```python
from build123d import *

# Parameters (mm, degrees)
SKETCH1_W            = 12
SKETCH1_H            = 23
BOSS_EXTRUDE1_DEPTH  = 6
SKETCH2_R            = 2.3
SKETCH2_R_2          = 4
CUT_EXTRUDE1_DEPTH   = 6
TAPER_FILLET_SIZE    = 14
TAPER_FILLET_SIZE_2  = 5
TAPER_FILLET2_SIZE   = 14
TAPER_FILLET2_SIZE_2 = 5
EDGE_FILLETS_R       = 1


with BuildPart() as part:
    # Sketch1 → Boss-Extrude1 (new body)
    with BuildSketch(Plane.XY):
        with Locations((6, 11.5)):
            Rectangle(SKETCH1_W, SKETCH1_H)
    extrude(amount=BOSS_EXTRUDE1_DEPTH)

    # Sketch2 → Cut-Extrude1 (cut)
    with BuildSketch(Plane.XY.offset(6)):
        with Locations((6, 18.5)):
            Circle(SKETCH2_R)
        with Locations((6, 6.5)):
            Circle(SKETCH2_R_2)
    extrude(amount=-CUT_EXTRUDE1_DEPTH, mode=Mode.SUBTRACT)

    # taper_fillet
    # an asymmetric fillet: 14, 5 mm, written as the material it takes off along each edge
    with BuildSketch(Plane(origin=(0, 23, -35), x_dir=(0, -1, 0), z_dir=(0, 0, 1))) as taper_fillet_piece_1:
        with BuildLine():
            Bezier((TAPER_FILLET_SIZE, 0), (0, 0), (0, TAPER_FILLET_SIZE_2), weights=[1, 0.707106781, 1])
            Line((0, TAPER_FILLET_SIZE_2), (0, 0))
            Line((0, 0), (TAPER_FILLET_SIZE, 0))
        make_face()
    extrude(amount=76, mode=Mode.SUBTRACT)

    # taper_fillet2
    # an asymmetric fillet: 14, 5 mm, written as the material it takes off along each edge
    with BuildSketch(Plane(origin=(12, 23, -35), x_dir=(0, -1, 0), z_dir=(0, 0, 1))) as taper_fillet2_piece_1:
        with BuildLine():
            Bezier((TAPER_FILLET2_SIZE, 0), (0, 0), (0, -TAPER_FILLET2_SIZE_2), weights=[1, 0.707106781, 1])
            Line((0, -TAPER_FILLET2_SIZE_2), (0, 0))
            Line((0, 0), (TAPER_FILLET2_SIZE, 0))
        make_face()
    extrude(amount=76, mode=Mode.SUBTRACT)

    # edge_fillets
    edge_fillets_edges = [part.edges().sort_by_distance(p)[0] for p in [
        (0, 4.5, 0),
        (0.853211897, 16.822053684, 0),
        (6, 23, 0),
        (12, 4.5, 0),
        (12, 4.5, 6),
        (0, 4.5, 6),
        (0.853211897, 16.822053684, 6),
        (6, 23, 6),
        (0, 0, 3),
        (6, 0, 6),
        (12, 0, 3),
        (6, 0, 0),
        (11.146788103, 16.822053684, 0),
        (11.146788103, 16.822053684, 6),
    ]]
    fillet(edge_fillets_edges, radius=EDGE_FILLETS_R)


solid = part.part
```
Model file for the job. Use its own axes, mm. Round coordinates to 2 decimals unless told otherwise and drop trailing zeros. Write each loop counter-clockwise with the first axis right and the second up, starting at its lowest first coordinate (ties: lowest second). Pieces come first, ordered by that corner, then holes. Notation, with made-up numbers: (87.25, -38.75) - (97.25, -38.75) arc R19 ccw to (97.25, -1.75) - close; hole circle Ø6 at (61.5, 19.25). An arc over 180 degrees is marked (long way). One line per item, written item: value.
(1) Drop a flat-ended pin along its axis: P1, Ø1.5, axis at y = 16, z = 3, coming from the +X side. Give the stop position or say it passes through.
Values follow:
P1: stops at x = 11.47
(2) Cut at B-B, the plane y = 6.5. Give the cut face in (x, z).
Values follow:
outline: (0, 1) arc R1 ccw to (1, 0) - (2, 0) - (2, 6) - (1, 6) arc R1 ccw to (0, 5) - close; (10, 0) - (11, 0) arc R1 ccw to (12, 1) - (12, 5) arc R1 ccw to (11, 6) - (10, 6) - close
(3) Cut at C-C, the plane z = 3. Give the number of separate pieces and of enclosed holes in the cut face, plus the area to 3 significant figures.
Values follow:
separate pieces: 1
enclosed holes: 2
area: 179 mm²
(4) Cut at A-A, the plane x = 6. Give the cut face in (y, z).
Values follow:
outline: (0, 1) arc R1 ccw to (1, 0) - (2.5, 0) - (2.5, 6) - (1, 6) arc R1 ccw to (0, 5) - close; (10.5, 0) - (16.2, 0) - (16.2, 6) - (10.5, 6) - close; (20.8, 0) - (22, 0) arc R1 ccw to (23, 1) - (23, 5) arc R1 ccw to (22, 6) - (20.8, 6) - close
(5) Wall check: probe 1 along Y at (x, z) = (6, 2.3); probe 2 along Y at (x, z) = (4, 5); probe 3 along X at (y, z) = (17, 3.75). Give the ranges that are in metal, low to high.
Values follow:
probe 1: y = 0 to 2.5, 10.5 to 16.2, 20.8 to 23
probe 2: y = 0 to 3.04, 9.96 to 17.36, 19.64 to 22.72
probe 3: x = 0.9 to 4.26, 7.74 to 11.1
(6) Two-plate mould, pull along X, no slides. Class faces 1 (the cylindrical face through (11.715, 4.944, 0.301)), 2 (the cylindrical face through (0.285, 5.056, 0.301)), 3 (the flat face through (6, 23, 3)), 4 (the cylindrical face through (5.133, 2.595, 3.042)): pulls with the +X half, pulls with the -X half, needs draft (parallel to the pull), parting line crosses it, or undercut.
Values follow:
face 1: pulls with the +X half
face 2: pulls with the -X half
face 3: needs draft
face 4: undercut
